Could you check a few things on this model? Use its own coordinates, in mm. A direction names the side the tool comes from. Coordinates: 2 decimals unless noted, no trailing zeros. Write each loop counter-clockwise with the first axis right and the second up, starting at its lowest first coordinate (ties: lowest second). Pieces come first, ordered by that corner, then holes.
```python
from build123d import *

# Parameters (mm, degrees)
SKETCH1_W           = 63.5
SKETCH1_H           = 190.5
BOSS_EXTRUDE1_DEPTH = 3.175
SKETCH3_R           = 2.0828
CUT_EXTRUDE2_DEPTH  = 526.850378691
SKETCH4_R           = 2.0828
CUT_EXTRUDE4_DEPTH  = 526.850378691
FILLET2_R           = 3.175


with BuildPart() as part:
    # Sketch1 → Boss-Extrude1 (new body)
    with BuildSketch(Plane(origin=(0, 0, 0), x_dir=(1, 0, 0), z_dir=(0, 1, 0))):
        Polygon((-242.686835374, -133.432512515), (-242.686835374, -385.491221995), (-242.686835374, -387.371651362), (-191.886835374, -438.171651362), (239.913164626, -438.171651362), (290.713164626, -387.371651362), (290.713164626, -133.371651362), (176.413164626, -82.571651362), (176.413164626, -133.371651362), (74.813164626, -196.871651362), (-26.786835374, -196.871651362), (-128.386835374, -133.371651362), (-128.386835374, -82.571651362), (-242.686835374, -133.371651362), align=None)
        with Locations((233.563164626, -243.80020948)):
            Rectangle(SKETCH1_W, SKETCH1_H, mode=Mode.SUBTRACT)
        with Locations((-185.536835374, -243.80020948)):
            Rectangle(SKETCH1_W, SKETCH1_H, mode=Mode.SUBTRACT)
    extrude(amount=BOSS_EXTRUDE1_DEPTH)

    # Sketch3 → Cut-Extrude2 (cut, through all)
    with BuildSketch(Plane(origin=(0, 0, 0), x_dir=(1, 0, 0), z_dir=(0, 1, 0))):
        with Locations(Location((-114.278235374, -270.125471314, 0), (0, 0, 270))):
            Circle(SKETCH3_R)
        with Locations(Location((-143.449035374, -284.13540948, 0), (0, 0, 270))):
            Circle(SKETCH3_R)
        with Locations(Location((-114.278235374, -217.474947647, 0), (0, 0, 270))):
            Circle(SKETCH3_R)
        with Locations(Location((-143.449035374, -203.46500948, 0), (0, 0, 270))):
            Circle(SKETCH3_R)
        with Locations(Location((191.475364626, -284.13540948, 0), (0, 0, 270))):
            Circle(SKETCH3_R)
        with Locations(Location((162.304564626, -270.125471314, 0), (0, 0, 270))):
            Circle(SKETCH3_R)
        with Locations(Location((162.304564626, -217.474947647, 0), (0, 0, 270))):
            Circle(SKETCH3_R)
        with Locations(Location((191.475364626, -203.46500948, 0), (0, 0, 270))):
            Circle(SKETCH3_R)
    extrude(amount=CUT_EXTRUDE2_DEPTH, mode=Mode.SUBTRACT)

    # Sketch4 → Cut-Extrude4 (cut, through all)
    with BuildSketch(Plane(origin=(0, 0, 0), x_dir=(1, 0, 0), z_dir=(0, 1, 0))):
        with Locations(Location((111.325664626, -210.298576853, 0), (0, 0, 270))):
            Circle(SKETCH4_R)
        with Locations(Location((111.325664626, -413.498576853, 0), (0, 0, 270))):
            Circle(SKETCH4_R)
        with Locations(Location((-63.299335374, -413.498576853, 0), (0, 0, 90))):
            Circle(SKETCH4_R)
        with Locations(Location((-63.299335374, -210.298576853, 0), (0, 0, 90))):
            Circle(SKETCH4_R)
        with BuildLine():
            Line((-50.599335374, -216.648576853), (98.625664626, -216.648576853))
            Line((98.625664626, -216.648576853), (98.625664626, -232.523576853))
            ThreePointArc((98.625664626, -232.523576853), (108.150664626, -242.048576853), (98.625664626, -251.573576853))
            Line((98.625664626, -251.573576853), (98.625664626, -384.923576853))
            ThreePointArc((98.625664626, -384.923576853), (108.150664626, -394.448576853), (98.625664626, -403.973576853))
            Line((98.625664626, -403.973576853), (98.625664626, -419.848576853))
            Line((98.625664626, -419.848576853), (-50.599335374, -419.848576853))
            Line((-50.599335374, -419.848576853), (-50.599335374, -403.973576853))
            ThreePointArc((-50.599335374, -403.973576853), (-60.124335374, -394.448576853), (-50.599335374, -384.923576853))
            Line((-50.599335374, -384.923576853), (-50.599335374, -251.573576853))
            ThreePointArc((-50.599335374, -251.573576853), (-60.124335374, -242.048576853), (-50.599335374, -232.523576853))
            Line((-50.599335374, -232.523576853), (-50.599335374, -216.648576853))
        make_face()
    extrude(amount=CUT_EXTRUDE4_DEPTH, mode=Mode.SUBTRACT)

    # Fillet2
    fillet2_edges = [part.edges().sort_by_distance(p)[0] for p in [
        (98.625664626, 1.5875, 419.848576853),
        (98.625664626, 1.5875, 216.648576853),
        (-50.599335374, 1.5875, 216.648576853),
        (-50.599335374, 1.5875, 419.848576853),
    ]]
    fillet(fillet2_edges, radius=FILLET2_R)


solid = part.part
```
1. I want a section at B-B on x = 0. Please give me the cut outline in (y, z) (3 decimals).
Verdict:
outline: (0, 196.872) - (3.175, 196.872) - (3.175, 216.649) - (0, 216.649) - close; (0, 419.849) - (3.175, 419.849) - (3.175, 438.172) - (0, 438.172) - close
2. If we mould it in two halves opening along X, with no side actions, what happens to faces 3 (the face through (139, 0, 297)), 4 (the face through (234.363, 1.565, 108.327)), 5 (the face through (-184.7, 1.6, 107.6)), 6 (the face through (-76.876, 1.565, 165.566))? For each: pulls with the +X half, pulls with the -X half, needs draft (parallel to the pull), parting line crosses it, or undercut.
Verdict:
face 3: needs draft
face 4: pulls with the +X half
face 5: pulls with the -X half
face 6: undercut
3. For pin 1 (1 mm diameter, centred on x = -88, y = 2, fed in from -Z); pin 2 (3.5 mm diameter, centred on x = 162.3, z = 217.47, fed in from -Y), each with a flat end and sliding along its axis, tell me the tip position at first contact or that it passes through.
Verdict:
pin 1: stops at z = 158.3
pin 2: passes through
4. I want a section at C-C on z = 361.5. Please give me the cut outline in (x, y) (3 decimals), plus the area to 3 significant figures.
Verdict:
outline: (-242.687, 0) - (-50.599, 0) - (-50.599, 3.175) - (-242.687, 3.175) - close; (98.626, 0) - (290.713, 0) - (290.713, 3.175) - (98.626, 3.175) - close
area: 1,220 mm2
5. I want a section at D-D on y = 1.8. Give the number of separate pieces and of enclosed holes in the cut face, plus the area to 3 significant figures.
Verdict:
separate pieces: 1
enclosed holes: 15
area: 97,700 mm2
6. I want a section at A-A on z = 324.5. Please give me the cut outline in (x, y) (3 decimals), plus the area to 3 significant figures.
Verdict:
outline: (-242.687, 0) - (-217.287, 0) - (-217.287, 3.175) - (-242.687, 3.175) - close; (-153.787, 0) - (-50.599, 0) - (-50.599, 3.175) - (-153.787, 3.175) - close; (98.626, 0) - (201.813, 0) - (201.813, 3.175) - (98.626, 3.175) - close; (265.313, 0) - (290.713, 0) - (290.713, 3.175) - (265.313, 3.175) - close
area: 817 mm2
7. Please list where these lines run through material, in increasing order: line 1 along X through (y, z) = (2.55, 352); line 2 along X through (y, z) = (2.7, 156); line 3 along X through (y, z) = (1.5, 279).
Verdict:
line 1: x = -242.69 to -50.6, 98.63 to 290.71
line 2: x = -242.69 to -217.29, -153.79 to -92.18, 140.21 to 201.81, 265.31 to 290.71
line 3: x = -242.69 to -217.29, -153.79 to -50.6, 98.63 to 201.81, 265.31 to 290.71
8. On a 3-axis mill with a long thin cutter (end or side, diameter ignored), from which of +Z, -Z, +X, -X, +Y, -Y can I reach the whole of each face in a straight line? I mean faces 1 (the face through (-217.64, 1.57, 412.42)), 2 (the face through (126.32, 1.57, 164.68)). Say none if no direction works.
Verdict:
face 1: +Z, -X, +Y, -Y
face 2: -Z, +Y, -Y
